Work out the finished part from the listing and answer in its coordinate system (mm). Coordinates: 2 decimals unless noted, no trailing zeros. Write each loop counter-clockwise with the first axis right and the second up, starting at its lowest first coordinate (ties: lowest second). Pieces come first, ordered by that corner, then holes. Notation, with made-up numbers: (30.5, 49.25) - (70.5, 49.25) arc R20 ccw to (70.5, 63.25) - close; hole circle Ø1 at (46, 52.25). An arc over 180 degrees is marked (long way). Answer as a JSON object with one key per item and string values. Group by question number.
from build123d import *

# Parameters (mm, degrees)
SKETCH1_R           = 62.5
BOSS_EXTRUDE1_DEPTH = 3
CUT_EXTRUDE5_DEPTH  = 89.439244682
CIRPATTERN4_COUNT   = 6
CUT_EXTRUDE6_DEPTH  = 89.439244682
FILLET1_R           = 10
FILLET2_R           = 1


with BuildPart() as part:
    # Sketch1 → Boss-Extrude1 (new body)
    with BuildSketch(Plane(origin=(0, 0, 0), x_dir=(0, 0, -1), z_dir=(1, 0, 0))):
        Circle(SKETCH1_R)
    extrude(amount=BOSS_EXTRUDE1_DEPTH)

    # Sketch6 → Cut-Extrude5 (cut, through all)
    with BuildSketch(Plane.ZY):
        with BuildLine():
            Line((-3, 54.918120871), (-3, 12.1346611))
            ThreePointArc((-3, 12.1346611), (-6.25, 10.825317547), (-9.008924778, 8.665406761))
            Line((-9.008924778, 8.665406761), (-46.060487802, 30.057136647))
            ThreePointArc((-46.060487802, 30.057136647), (-27.5, 47.631397208), (-3, 54.918120871))
        make_face()
    cut_extrude5 = extrude(amount=-CUT_EXTRUDE5_DEPTH, mode=Mode.SUBTRACT)

    # CirPattern4: Cut-Extrude5 ×6 about axis
    cirpattern4_axis = Axis((0, 0, 0), (1, 0, 0))
    for i in range(1, CIRPATTERN4_COUNT):
        add(cut_extrude5.rotate(cirpattern4_axis, i * 360 / CIRPATTERN4_COUNT), mode=Mode.SUBTRACT)

    # Sketch7 → Cut-Extrude6 (cut, through all)
    with BuildSketch(Plane.ZY):
        Polygon((0, 3.960622847), (-3.43, 1.980311423), (-3.43, -1.980311423), (0, -3.960622847), (3.43, -1.980311423), (3.43, 1.980311423), align=None)
    extrude(amount=-CUT_EXTRUDE6_DEPTH, mode=Mode.SUBTRACT)

    # Fillet1
    # the kernel refuses this fillet: 10 mm, written as the material it adds along each edge
    with BuildSketch(Plane(origin=(0, 12.1346611, 3), x_dir=(0, 1, 0), z_dir=(1, 0, 0)), Plane(origin=(0, 3.469254338, 12.008924778), x_dir=(0, 0.5000000000000027, 0.8660254037844372), z_dir=(1, 0, 0)), Plane(origin=(0, -8.665406761, 9.008924778), x_dir=(0, -0.4999999999999975, 0.8660254037844402), z_dir=(1, 0, 0)), Plane(origin=(0, -12.1346611, -3), x_dir=(0, -1, 0), z_dir=(1, 0, 0)), Plane(origin=(0, -3.469254338, -12.008924778), x_dir=(0, -0.500000000000002, -0.8660254037844375), z_dir=(1, 0, 0)), Plane(origin=(0, 8.665406761, -9.008924778), x_dir=(0, 0.4999999999999975, -0.86602540378444), z_dir=(1, 0, 0))) as fillet1_piece_1:
        with BuildLine():
            CenterArc((6.229706573, 10), FILLET1_R, 215.294394677, 54.705605323)
            ThreePointArc((-1.932234615, 4.222222222), (-0.768344169, 2.201618925), (0, 0))
            Line((0, 0), (6.229706573, 0))
        make_face()
    extrude(amount=3)
    with BuildSketch(Plane(origin=(0, 8.665406761, 9.008924778), x_dir=(0, 0.5000000000000008, 0.8660254037844382), z_dir=(1, 0, 0)), Plane(origin=(0, -3.469254338, 12.008924778), x_dir=(0, -0.49999999999999983, 0.8660254037844387), z_dir=(1, 0, 0)), Plane(origin=(0, -12.1346611, 3), x_dir=(0, -1, 0), z_dir=(1, 0, 0)), Plane(origin=(0, -8.665406761, -9.008924778), x_dir=(0, -0.5000000000000001, -0.8660254037844385), z_dir=(1, 0, 0)), Plane(origin=(0, 3.469254338, -12.008924778), x_dir=(0, 0.5000000000000001, -0.8660254037844385), z_dir=(1, 0, 0)), Plane(origin=(0, 12.1346611, -3), x_dir=(0, 1, 0), z_dir=(1, 0, 0))) as fillet1_piece_2:
        with BuildLine():
            CenterArc((6.229706573, -10), FILLET1_R, 90, 54.705605323)
            ThreePointArc((-1.932234615, -4.222222222), (-0.768344169, -2.201618925), (0, 0))
            Line((0, 0), (6.229706573, 0))
        make_face()
    extrude(amount=3)

    # Fillet2
    fillet2_edges = [part.edges().sort_by_distance(p)[0] for p in [
        (1.5, 54.918120871, -3),
        (1.5, -54.918120871, -3),
        (1.5, -30.057136647, -46.060487802),
        (1.5, -30.057136647, 46.060487802),
        (1.5, -54.918120871, 3),
        (1.5, 54.918120871, 3),
        (1.5, 30.057136647, 46.060487802),
        (1.5, 24.860984224, 49.060487802),
        (1.5, -24.860984224, 49.060487802),
        (1.5, -24.860984224, -49.060487802),
        (1.5, 24.860984224, -49.060487802),
        (1.5, 30.057136647, -46.060487802),
    ]]
    fillet(fillet2_edges, radius=FILLET2_R)


solid = part.part
Q1. Section D-D on y = -39 is taken. Determine the outline of the cut face in (x, z), plus the area to 3 significant figures.
Q2. Flat-ended cylindrical pins translate along their axes: pin 1 Ø1.5 at (x, y) = (1.5, -40.5) entering from +Z; pin 2 Ø1.5 at (x, y) = (2, 33) entering from +Z; pin 3 Ø0.9 at (x, y) = (1.5, -30.5) entering from -Z. Find the tip coordinate at first contact, or state that the pin passes through.
Q3. For a pull along Z with two mould halves and no side action, classify faces 1 (the face through (1.48, 2.75, 62.44)), 2 (the face through (1, -36, 3)) as +Z half, -Z half, draft (parallel to the pull), parting line (faces both ways), or undercut.
Q4. Consider L1, parallel to Z at x = 1.3, y = -5; L2, parallel to Z at x = 2.05, y = -9.5; L3, parallel to Y at x = 2.1, z = -29. Determine where each line is inside the solid, lowest interval first. Write a range as from..to.
Q5. Section B-B on y = 38 is taken. Determine the outline of the cut face in (x, z), plus the area to 3 significant figures.
Q6. Section A-A on z = 43 is taken. Determine the outline of the cut face in (x, y).
Q7. Section C-C on x = 1.15 is taken. Count the separate pieces of the cut face and the enclosed holes in it, plus the area to 3 significant figures.
Numbers:
{
 "1": {"outline": "(0, -48.84) - (3, -48.84) - (3, -38.78) - (0, -38.78) - close; (0, -3) - (3, -3) - (3, 3) - (0, 3) - close; (0, 38.78) - (3, 38.78) - (3, 48.84) - (0, 48.84) - close", "area": "78.3 mm²"},
 "2": {"pin 1": "stops at z = 48.23", "pin 2": "stops at z = 53.54", "pin 3": "stops at z = -54.8"},
 "3": {"face 1": "parting line", "face 2": "undercut"},
 "4": {"L1": "z = -62.3..-54.77, -15.34..15.34, 54.77..62.3", "L2": "z = -61.77..-54.17, -22.45..22.45, 54.17..61.77", "L3": "y = -55.36..-46.73, -20.21..-13.28, 13.28..20.21, 46.73..55.36"},
 "5": {"outline": "(0, -49.62) - (3, -49.62) - (3, -39.76) - (0, -39.76) - close; (0, -3) - (3, -3) - (3, 3) - (0, 3) - close; (0, 39.76) - (3, 39.76) - (3, 49.62) - (0, 49.62) - close", "area": "77.2 mm²"},
 "6": {"outline": "(0, -45.36) - (3, -45.36) - (3, -34.29) - (0, -34.29) - close; (0, -28.29) - (3, -28.29) - (3, -21.36) - (0, -21.36) - close; (0, 21.36) - (3, 21.36) - (3, 28.29) - (0, 28.29) - close; (0, 34.29) - (3, 34.29) - (3, 45.36) - (0, 45.36) - close"},
 "7": {"separate pieces": "1", "enclosed holes": "7", "area": "4,820 mm²"}
}
